```python
from build123d import *

# Parameters (mm, degrees)
F0_W     = 3.175
F0_H     = 38.1
F1_DEPTH = 22.225
F0_W_2   = 38.1
F0_R     = 11.1125
F2_DEPTH = 3.175
F4_D     = 4.4958
F5_D     = 4.4958
F6_D     = 4.4958
F7_D     = 4.4958
F8_D     = 4.4958
F9_D     = 4.4958


with BuildPart() as f1:
    # F0 (on Top) → F1 (new body)
    with BuildSketch(Plane.XY):
        with Locations((19.05, 0)):
            Rectangle(F0_W, F0_H)
    extrude(amount=F1_DEPTH)

    # F0 (on Top) → F2 (join)
    with BuildSketch(Plane.XY):
        with Locations((-1.5875, 0)):
            Rectangle(F0_W_2, F0_H)
        with Locations((-1.5875, 0)):
            Circle(F0_R, mode=Mode.SUBTRACT)
    extrude(amount=F2_DEPTH)

    # F4 (through all)
    with Locations(Plane(origin=(0, 0, 0), x_dir=(1, 0, 0), z_dir=(0, 0, -1))):
        with Locations((-15.0622, 13.4747)):
            Hole(F4_D / 2)

    # F5 (through all)
    with Locations(Plane(origin=(0, 0, 0), x_dir=(1, 0, 0), z_dir=(0, 0, -1))):
        with Locations((-15.0622, -13.4747)):
            Hole(F5_D / 2)

    # F6 (through all)
    with Locations(Plane(origin=(0, 0, 0), x_dir=(1, 0, 0), z_dir=(0, 0, -1))):
        with Locations((11.8872, -13.4747)):
            Hole(F6_D / 2)

    # F7 (through all)
    with Locations(Plane(origin=(0, 0, 0), x_dir=(1, 0, 0), z_dir=(0, 0, -1))):
        with Locations((11.8872, 13.4747)):
            Hole(F7_D / 2)

    # F8 (through all)
    with Locations(Plane(origin=(17.4625, 0, 0), x_dir=(0, -1, 0), z_dir=(-1, 0, 0))):
        with Locations((-13.4747, 12.7)):
            Hole(F8_D / 2)

    # F9 (through all)
    with Locations(Plane(origin=(17.4625, 0, 0), x_dir=(0, -1, 0), z_dir=(-1, 0, 0))):
        with Locations((13.4747, 12.7)):
            Hole(F9_D / 2)


solid = f1.part
```
Geometry: final body of the model. Coordinates: model frame, mm. A direction names the side the tool comes from. Coordinates: 2 decimals unless noted, no trailing zeros. Order: outer loops, then holes, each group sorted by start corner. A loop starts at its lowest first (then second) coordinate and runs counter-clockwise, first axis right, second up. Notation, with made-up numbers: (6, 73) - (10, 73) arc R20 cw to (10, 103) - close; hole circle Ø9 at (-15, -6.5). An arc over 180 degrees is marked (long way). Return JSON: item names as keys, results as strings. Group by question number.
1. Pin query (flat end, axial travel): pin 1 (5 mm diameter, centred on y = -13.47, z = 12.7, fed in from -X); pin 2 (7 mm diameter, centred on x = -15.06, y = 13.47, fed in from +Z) (3 decimals). Return the tip coordinate at first contact, or that it passes through.
2. Cut plane D-D (y = 12). Output: boundary loops of the cut face in (x, z) (1 decimal).
3. Cut plane B-B (y = 0). Output: boundary loops of the cut face in (x, z) (1 decimal), plus the area to 3 significant figures.
4. Pull-direction query (X, two-part tool) for faces 1 (the face through (17.463, 0, 13)), 2 (the face through (-13.278, -12.107, 1.61)), 3 (the face through (19.072, -11.331, 13.375)); classes: pulls with the +X half, pulls with the -X half, needs draft (parallel to the pull), parting line crosses it, or undercut.
5. Material intervals for line 1 along Z through (x, y) = (16.5, 3.5) (3 decimals); line 2 along X through (y, z) = (-16.5, 17.25); line 3 along Y through (x, z) = (2, 2.5), sorted ascending. Write a range as [from, to].
6. Cut plane A-A (z = 12.7). Output: boundary loops of the cut face in (x, y).
7. Set-up query: faces 4 (the face through (9, 5, 0)), 5 (the face through (7, 9, 3.175)). Return all of +Z, -Z, +X, -X, +Y, -Y with unobstructed straight access to the full face (end or side cutting, diameter ignored); none if empty.
8. Cut plane C-C (x = 12). Output: boundary loops of the cut face in (y, z) (3 decimals).
Resolved:
{
 "1": {"pin 1": "stops at x = 17.46", "pin 2": "stops at z = 3.175"},
 "2": {"outline": "(-20.6, 0) - (-16.8, 0) - (-16.8, 3.2) - (-20.6, 3.2) - close; (-13.4, 0) - (10.2, 0) - (10.2, 3.2) - (-13.4, 3.2) - close; (13.6, 0) - (20.6, 0) - (20.6, 11) - (17.5, 11) - (17.5, 3.2) - (13.6, 3.2) - close; (17.5, 14.4) - (20.6, 14.4) - (20.6, 22.2) - (17.5, 22.2) - close"},
 "3": {"outline": "(-20.6, 0) - (-12.7, 0) - (-12.7, 3.2) - (-20.6, 3.2) - close; (9.5, 0) - (20.6, 0) - (20.6, 22.2) - (17.5, 22.2) - (17.5, 3.2) - (9.5, 3.2) - close", "area": "121 mm²"},
 "4": {"face 1": "pulls with the -X half", "face 2": "undercut", "face 3": "needs draft"},
 "5": {"line 1": "z = [0, 3.175]", "line 2": "x = [17.46, 20.64]", "line 3": "y = [-19.05, -10.52], [10.52, 19.05]"},
 "6": {"outline": "(17.46, -19.05) - (20.64, -19.05) - (20.64, -15.72) - (17.46, -15.72) - close; (17.46, -11.23) - (20.64, -11.23) - (20.64, 11.23) - (17.46, 11.23) - close; (17.46, 15.72) - (20.64, 15.72) - (20.64, 19.05) - (17.46, 19.05) - close"},
 "7": {"face 4": "-Z, +X, -X, +Y, -Y", "face 5": "+Z, -X, +Y, -Y"},
 "8": {"outline": "(-19.05, 0) - (-15.72, 0) - (-15.72, 3.175) - (-19.05, 3.175) - close; (-11.23, 0) - (11.23, 0) - (11.23, 3.175) - (-11.23, 3.175) - close; (15.72, 0) - (19.05, 0) - (19.05, 3.175) - (15.72, 3.175) - close"}
}
